For this review, take the finished solid that the model builds, in its own axes (mm). A direction names the side the tool comes from. Round coordinates to 2 decimals unless told otherwise and drop trailing zeros. Write each loop counter-clockwise with the first axis right and the second up, starting at its lowest first coordinate (ties: lowest second). Pieces come first, ordered by that corner, then holes.
from build123d import *

# Parameters (mm, degrees)
SKETCH1_W           = 100
SKETCH1_H           = 100
BOSS_EXTRUDE1_DEPTH = 5
LPATTERN2_START     = -5
LPATTERN2_DEPTH     = 10


# Read off the part's stored shape, not the designer's step: LPattern2
with BuildPart() as part:
    # Sketch1 → Boss-Extrude1 (new, symmetric)
    with BuildSketch(Plane.XY):
        Rectangle(SKETCH1_W, SKETCH1_H)
        with BuildLine():
            Line((-38.686291501, -24.544155877), (-24.544155877, -38.686291501))
            ThreePointArc((-24.544155877, -38.686291501), (-24.544155877, -44.343145751), (-30.201010127, -44.343145751))
            Line((-30.201010127, -44.343145751), (-44.343145751, -30.201010127))
            ThreePointArc((-44.343145751, -30.201010127), (-44.343145751, -24.544155877), (-38.686291501, -24.544155877))
        make_face(mode=Mode.SUBTRACT)
    extrude(amount=BOSS_EXTRUDE1_DEPTH, both=True)

    # LPattern2 outline → LPattern2 (cut)
    with BuildSketch(Plane.XY.offset(LPATTERN2_START)):
        with BuildLine():
            Line((24.953318806, 10.811183182), (10.811183182, 24.953318806))
            ThreePointArc((10.811183182, 24.953318806), (5.154328933, 24.953318806), (5.154328933, 19.296464556))
            Line((5.154328933, 19.296464556), (19.296464556, 5.154328933))
            ThreePointArc((19.296464556, 5.154328933), (24.953318806, 5.154328933), (24.953318806, 10.811183182))
        make_face()
        with BuildLine():
            Line((15.053823869, 0.911688245), (0.911688245, 15.053823869))
            ThreePointArc((0.911688245, 15.053823869), (-4.745166004, 15.053823869), (-4.745166004, 9.39696962))
            Line((-4.745166004, 9.39696962), (9.39696962, -4.745166004))
            ThreePointArc((9.39696962, -4.745166004), (15.053823869, -4.745166004), (15.053823869, 0.911688245))
        make_face()
        with BuildLine():
            Line((5.154328933, -8.987806691), (-8.987806691, 5.154328933))
            ThreePointArc((-8.987806691, 5.154328933), (-14.644660941, 5.154328933), (-14.644660941, -0.502525317))
            Line((-14.644660941, -0.502525317), (-0.502525317, -14.644660941))
            ThreePointArc((-0.502525317, -14.644660941), (5.154328933, -14.644660941), (5.154328933, -8.987806691))
        make_face()
        with BuildLine():
            Line((-4.745166004, -18.887301628), (-18.887301628, -4.745166004))
            ThreePointArc((-18.887301628, -4.745166004), (-24.544155877, -4.745166004), (-24.544155877, -10.402020254))
            Line((-24.544155877, -10.402020254), (-10.402020254, -24.544155877))
            ThreePointArc((-10.402020254, -24.544155877), (-4.745166004, -24.544155877), (-4.745166004, -18.887301628))
        make_face()
        with BuildLine():
            Line((-14.644660941, -28.786796564), (-28.786796564, -14.644660941))
            ThreePointArc((-28.786796564, -14.644660941), (-34.443650813, -14.64466094), (-34.443650814, -20.30151519))
            Line((-34.443650814, -20.30151519), (-20.30151519, -34.443650814))
            ThreePointArc((-20.30151519, -34.443650814), (-14.64466094, -34.443650813), (-14.644660941, -28.786796564))
        make_face()
    extrude(amount=LPATTERN2_DEPTH, mode=Mode.SUBTRACT)


solid = part.part
(1) For faces 1 (the face through (-1.818, -2.016, -0.07)), 2 (the face through (50, -1, 0)), list the 3-axis set-ups (+Z, -Z, +X, -X, +Y, -Y) from which the entire face can be reached by the end or side of a thin tool; tool diameter is ignored.
Geometry check:
face 1: +Z, -Z
face 2: +Z, -Z, +X, +Y, -Y
(2) For line 1 along Y through (x, z) = (10, -4.25); line 2 along Y through (x, z) = (-23, 1.25); line 3 along X through (y, z) = (14.5, 0), list the stretches that pass through material, from the lowest coordinate up.
Geometry check:
line 1: y = -50 to -5.24, 5.97 to 14.45, 25.58 to 50
line 2: y = -50 to -31.75, -20.43 to -11.95, -3.79 to 50
line 3: x = -50 to -5.21, 1.47 to 9.95, 21.26 to 50
(3) We need section B-B, the plane x = -37.5. Give the boundary of the cut face in (y, z).
Geometry check:
outline: (-50, -5) - (-37.04, -5) - (-37.04, 5) - (-50, 5) - close; (-25.73, -5) - (50, -5) - (50, 5) - (-25.73, 5) - close
(4) Mouldability with a two-part tool opening along Y and no side actions: class faces 3 (the face through (-50, -1, 0)), 4 (the face through (-1, -50, 0)), 5 (the face through (5.1, -14.7, -0.1)) as pulls with the +Y half, pulls with the -Y half, needs draft (parallel to the pull), parting line crosses it, or undercut.
Geometry check:
face 3: needs draft
face 4: pulls with the -Y half
face 5: undercut
(5) We need section A-A, the plane z = 3. Give the boundary of the cut face in (x, y), and give its area (3 significant figures).
Geometry check:
outline: (-50, -50) - (50, -50) - (50, 50) - (-50, 50) - close; hole (-44.34, -30.2) - (-30.2, -44.34) arc R4 ccw to (-24.54, -38.69) - (-38.69, -24.54) arc R4 ccw to start; hole (-34.44, -20.3) - (-20.3, -34.44) arc R4 ccw to (-14.64, -28.79) - (-28.79, -14.64) arc R4 ccw to start; hole (-24.54, -10.4) - (-10.4, -24.54) arc R4 ccw to (-4.75, -18.89) - (-18.89, -4.75) arc R4 ccw to start; hole (-14.64, -0.5) - (-0.5, -14.64) arc R4 ccw to (5.15, -8.99) - (-8.99, 5.15) arc R4 ccw to start; hole (-4.75, 9.4) - (9.4, -4.75) arc R4 ccw to (15.05, 0.91) - (0.91, 15.05) arc R4 ccw to start; hole (5.15, 19.3) - (19.3, 5.15) arc R4 ccw to (24.95, 10.81) - (10.81, 24.95) arc R4 ccw to start
area: 8,740 mm2
